Could you check a few things on this model? Use its own coordinates, in mm. Round coordinates to 2 decimals unless told otherwise and drop trailing zeros. Loops run counter-clockwise (first coordinate to the right, second up) from the corner with the lowest first, then second, coordinate; pieces in that order, holes last. Notation, with made-up numbers: (-7.75, -14.5) -> (14.25, -14.5) arc R27 ccw to (14.25, 24.5) -> close; hole circle Ø8 at (45, -9). An arc over 180 degrees is marked (long way). Write each question's results on one line, items separated by ' | '. Start each with the question number.
1) If I drill on probe 1 along Y at (x, z) = (-32, 2.15); probe 2 along X at (y, z) = (-58, 3.6); probe 3 along Y at (x, z) = (-27, 2.35), over which ranges is the centre line in solid material (lowest first)?
2) For P1, Ø1.5, axis at x = 1.5, z = 3.5, coming from the -Y side; P2, Ø1.5, axis at y = -75.5, z = 3, coming from the +X side; P3, Ø2.5, axis at y = -74, z = 3, coming from the -X side; P4, Ø1, axis at x = -32, y = -23, coming from the -Z side, each with a flat end and sliding along its axis, tell me the tip position at first contact or that it passes through.
3) Imagine slicing it at A-A, the plane z = 1.3. List the corners of the cut face in (x, y) for me, plus the area to 3 significant figures.
4) Imagine slicing it at B-B, the plane y = -58. List the corners of the cut face in (x, z) for me, plus the area to 4 significant figures.
5) Imagine slicing it at C-C, the plane x = -32. List the corners of the cut face in (y, z) for me.
Autodesk Inventor part; units mm, degrees
ref_plane "YZ Plane" through (0, 0, 0) normal (1, 0, 0) x (0, 1, 0)
ref_plane "XZ Plane" through (0, 0, 0) normal (0, 1, 0) x (-1, 0, 0)
ref_plane "XY Plane" through (0, 0, 0) normal (0, 0, 1) x (1, 0, 0)
sketch "草图1" plane through (0, 0, 0) normal (0, 0, 1) x (1, 0, 0)
  line L0 (-30, 0) -> (-45, 0)
  line L1 (-30, 0) -> (-30, 5)
  line L2 (-45, 5) -> (-30, 5)
  line L3 (-45, 0) -> (-45, 5)
  line L4 (0, 0) -> (-15, 0)
  line L5 (0, 0) -> (0, 5)
  line L6 (-15, 5) -> (0, 5)
  line L7 (-15, 0) -> (-15, 5)
  line L8 (-42, -72) -> (-37, -72)
  line L9 (5, 0) -> (5, -12.0239)
  line L10 (5, 0) -> (-50, 0)
  line L11 (-50, 0) -> (-50, -72)
  line L12 (-50, -72) -> (5, -72)
  line L13 (5, -72) -> (5, 0)
  line L14 (-45, -72) -> (-30, -72)
  line L15 (-30, -72) -> (-30, -77)
  line L16 (-30, -77) -> (-45, -77)
  line L17 (-45, -77) -> (-45, -72)
  line L18 (-15, -72) -> (0, -72)
  line L19 (0, -72) -> (0, -77)
  line L20 (0, -77) -> (-15, -77)
  line L21 (-15, -77) -> (-15, -72)
  circle A0 centre (-32, -58) radius 0.85
  circle A1 centre (-32, -23) radius 0.85
  dimension "d0" = 55
  dimension "d1" = 5
  dimension "d2" = 1.7
  dimension "d3" = 14
  dimension "d4" = 37
  dimension "d5" = 1.7
  dimension "d6" = 35
  dimension "d7" = 18
extrude "拉伸1" add sketch "草图1" along normal blind 5
properties part number "drive-fix"
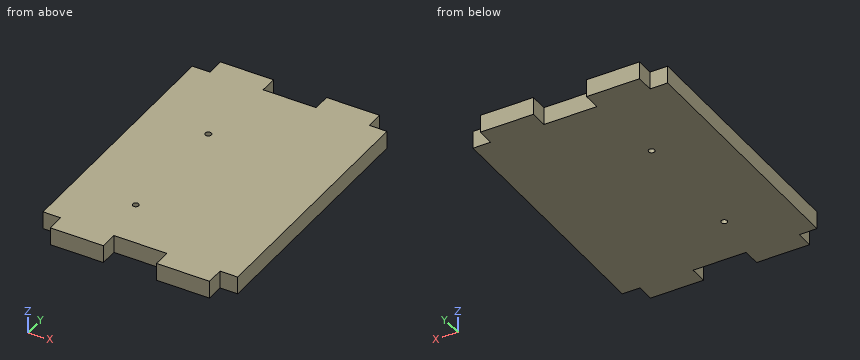
Checked values:
1) probe 1: -77 to -58.85, -57.15 to -23.85, -22.15 to 5 | probe 2: -50 to -32.85, -31.15 to 5 | probe 3: -72 to 0
2) P1: y = -72 | P2: x = 0 | P3: x = -45 | P4: through
3) outline: (-50, -72) -> (-45, -72) -> (-45, -77) -> (-30, -77) -> (-30, -72) -> (-15, -72) -> (-15, -77) -> (0, -77) -> (0, -72) -> (5, -72) -> (5, 0) -> (0, 0) -> (0, 5) -> (-15, 5) -> (-15, 0) -> (-30, 0) -> (-30, 5) -> (-45, 5) -> (-45, 0) -> (-50, 0) -> close; hole circle Ø1.7 at (-32, -58); hole circle Ø1.7 at (-32, -23) | area: 4,260 mm^2
4) outline: (-50, 0) -> (-32.85, 0) -> (-32.85, 5) -> (-50, 5) -> close; (-31.15, 0) -> (5, 0) -> (5, 5) -> (-31.15, 5) -> close | area: 266.5 mm^2
5) outline: (-77, 0) -> (-58.85, 0) -> (-58.85, 5) -> (-77, 5) -> close; (-57.15, 0) -> (-23.85, 0) -> (-23.85, 5) -> (-57.15, 5) -> close; (-22.15, 0) -> (5, 0) -> (5, 5) -> (-22.15, 5) -> close
